```python
from build123d import *

# Parameters (mm, degrees)
F1_DEPTH = 0.8
F3_DEPTH = 4
F5_DEPTH = 0.6


with BuildPart() as f1:
    # F0 (on Top) → F1 (new body)
    with BuildSketch(Plane.XY):
        with BuildLine():
            ThreePointArc((0, 7), (-2.12132, 6.12132), (-3, 4))
            Line((-3, 4), (-3, -4))
            ThreePointArc((-3, -4), (-2.12132, -6.12132), (0, -7))
            ThreePointArc((0, -7), (2.12132, -6.12132), (3, -4))
            Line((3, -4), (3, 4))
            ThreePointArc((3, 4), (2.12132, 6.12132), (0, 7))
        make_face()
    extrude(amount=F1_DEPTH)

    # F2 (on face) → F3 (join)
    with BuildSketch(Plane.XY.offset(0.8)):
        with BuildLine():
            ThreePointArc((0, 2), (-0.707107, 1.707107), (-1, 1))
            Line((-1, 1), (-1, -1))
            ThreePointArc((-1, -1), (-0.707107, -1.707107), (0, -2))
            ThreePointArc((0, -2), (0.707107, -1.707107), (1, -1))
            Line((1, -1), (1, 1))
            ThreePointArc((1, 1), (0.707107, 1.707107), (0, 2))
        make_face()
    extrude(amount=F3_DEPTH)

    # F4 (on face) → F5 (join)
    with BuildSketch(Plane.XY.offset(4.8)):
        with BuildLine():
            ThreePointArc((0, 4), (-1.414214, 3.414214), (-2, 2))
            Line((-2, 2), (-2, -2))
            ThreePointArc((-2, -2), (-1.414214, -3.414214), (0, -4))
            ThreePointArc((0, -4), (1.414214, -3.414214), (2, -2))
            Line((2, -2), (2, 2))
            ThreePointArc((2, 2), (1.414214, 3.414214), (0, 4))
        make_face()
    extrude(amount=F5_DEPTH)


solid = f1.part
```
Source: CAD feature listing. Evaluate the final solid. Frame: model axes, mm. A direction names the side the tool comes from. Round coordinates to 2 decimals unless told otherwise and drop trailing zeros. Loops run counter-clockwise (first coordinate to the right, second up) from the corner with the lowest first, then second, coordinate; pieces in that order, holes last.
1. Section query D-D on y = 5. Output: boundary loops of the cut face in (x, z).
2. Section query B-B on z = 5.05. Output: boundary loops of the cut face in (x, y).
3. Section query C-C on x = 0.85. Output: boundary loops of the cut face in (y, z), and give its area (3 significant figures).
4. Mould query, pull axis Z, two halves, no side actions, for faces 3 (the flat face through (1, 0, 3)), 4 (the flat face through (0, 0, 0)), 5 (the flat face through (-1.4, 0.1, 0.8)), 6 (the flat face through (0, 0, 5.4)). Classes: released by +Z, released by -Z, zero draft, split by the parting line, or undercut.
5. Section query A-A on x = -1.5. Output: boundary loops of the cut face in (y, z).
6. Access query for faces 1 (the flat face through (1.3, 0.1, 4.8)), 2 (the flat face through (-1, 0, 3)). Directions: +Z, -Z, +X, -X, +Y, -Y. A direction counts if a zero-diameter tool reaches every point of the face in a straight line with its end or side. Return the directions, or none.
7. Ray query, L1, parallel to Z at x = -1.15, y = 0.75; L2, parallel to X at y = -1, z = 3; L3, parallel to Z at x = -1.5, y = 5.25. Return the intervals inside material, ascending.
8. Contact query for flat-ended pins moving along their axis: pin 1 (2 mm diameter, centred on y = 0.5, z = 2, fed in from -X); pin 2 (0.7 mm diameter, centred on y = -0.5, z = 5, fed in from +X); pin 3 (0.5 mm diameter, centred on y = -0.5, z = 5, fed in from -X). Output: stop coordinate, or through.
Answers below:
1. outline: (-2.83, 0) - (2.83, 0) - (2.83, 0.8) - (-2.83, 0.8) - close
2. outline: (-2, -2) arc R2 ccw to (0, -4) arc R2 ccw to (2, -2) - (2, 2) arc R2 ccw to (0, 4) arc R2 ccw to (-2, 2) - close
3. outline: (-6.88, 0) - (6.88, 0) - (6.88, 0.8) - (1.53, 0.8) - (1.53, 4.8) - (3.81, 4.8) - (3.81, 5.4) - (-3.81, 5.4) - (-3.81, 4.8) - (-1.53, 4.8) - (-1.53, 0.8) - (-6.88, 0.8) - close
3. area: 27.8 mm2
4. face 3: undercut
4. face 4: released by -Z
4. face 5: undercut
4. face 6: released by +Z
5. outline: (-6.6, 0) - (6.6, 0) - (6.6, 0.8) - (-6.6, 0.8) - close; (-3.32, 4.8) - (3.32, 4.8) - (3.32, 5.4) - (-3.32, 5.4) - close
6. face 1: none
6. face 2: -X, +Y, -Y
7. L1: z = 0 to 0.8, 4.8 to 5.4
7. L2: x = -1 to 1
7. L3: z = 0 to 0.8
8. pin 1: stops at x = -1
8. pin 2: stops at x = 2
8. pin 3: stops at x = -2
